Design review of the part built by this model. Coordinates are the model's own, in mm. A direction names the side the tool comes from. Round coordinates to 2 decimals unless told otherwise and drop trailing zeros. Loops run counter-clockwise (first coordinate to the right, second up) from the corner with the lowest first, then second, coordinate; pieces in that order, holes last. Notation, with made-up numbers: (7.25, 59) - (11.25, 59) arc R12 cw to (11.25, 69) - close; hole circle Ø1 at (43, 55). An arc over 180 degrees is marked (long way). Return JSON: item names as keys, results as strings. Group by question number.
(1) Clearance check with flat-ended pins moving along their axes: pin 1 (6 mm diameter, centred on x = -9.98, z = -5.76, fed in from +Y); pin 2 (1.6 mm diameter, centred on x = 9.99, z = 5.76, fed in from -Y); pin 3 (2 mm diameter, centred on x = 0, z = 11.53, fed in from +Y); pin 4 (5 mm diameter, centred on x = 2, z = -4.5, fed in from -Y). State where each tip first meets the part, or that it passes through.
(2) Wall thickness on L1, parallel to X at y = -1.35, z = 0; L2, parallel to X at y = -0.2, z = 5.75; L3, parallel to X at y = -1.55, z = 6: over which ranges is each line inside the solid? List them lowest first. Write a range as [from, to].
(3) For faces 5 (the cylindrical face through (0.709, 1.232, 9.816)), 6 (the cylindrical face through (-2.91, 0.13, -7.02)), 7 (the cylindrical face through (0.27, -0.81, 10.67)), list the 3-axis set-ups (+Z, -Z, +X, -X, +Y, -Y) from which the entire face can be reached by the end or side of a thin tool; tool diameter is ignored.
(4) The part is to be moulded in two halves that separate along Z. For faces 1 (the cylindrical face through (9.1, -0.8, -5.6)), 2 (the cylindrical face through (-9.1, -0.8, -5.6)), 3 (the cylindrical face through (0.66, 0.421, 14.985)), 4 (the flat face through (-3.5, 2.7, -6.4)), say which applies: pulls with the +Z half, pulls with the -Z half, needs draft (parallel to the pull), parting line crosses it, or undercut.
(5) We need section A-A, the plane y = -1.2. Write out the cut boundary in (x, z) (3 decimals).
(6) We need section B-B, the plane x = 0. Give the number of separate pieces and of enclosed holes in the cut face, and give its area (3 significant figures).
from build123d import *

# Parameters (mm, degrees)
SKETCH_1_R          = 15
SKETCH_1_R_2        = 7.1
SKETCH_1_R_3        = 1.85
EXTRUDE_1_DEPTH     = 2.7
EXTRUDE_START       = 1.8
SKETCH_2_R          = 15
SKETCH_2_R_2        = 7.1
SKETCH_2_R_3        = 0.9
EXTRUDE_2_DEPTH     = 1.8
SKETCH_3_R          = 7.6
CUT_EXTRUDE_1_DEPTH = 4.1
CHAMFER_1_SIZE      = 0.2
CHAMFER_2_SIZE      = 0.4


with BuildPart() as part:
    # 草图1 → 凸台-拉伸1 (new body)
    with BuildSketch(Plane(origin=(0, 0, 0), x_dir=(1, 0, 0), z_dir=(0, 1, 0))):
        with Locations(Location((0, 0, 0), (0, 0, 90))):
            Circle(SKETCH_1_R)
        with Locations(Location((0, 0, 0), (0, 0, 90))):
            Circle(SKETCH_1_R_2, mode=Mode.SUBTRACT)
        with Locations(Location((0, 11.525, 0), (0, 0, 90))):
            Circle(SKETCH_1_R_3, mode=Mode.SUBTRACT)
        with Locations(Location((9.980942779, 5.7625, 0), (0, 0, 90))):
            Circle(SKETCH_1_R_3, mode=Mode.SUBTRACT)
        with Locations(Location((9.980942779, -5.7625, 0), (0, 0, 90))):
            Circle(SKETCH_1_R_3, mode=Mode.SUBTRACT)
        with Locations(Location((0, -11.525, 0), (0, 0, 90))):
            Circle(SKETCH_1_R_3, mode=Mode.SUBTRACT)
        with Locations(Location((-9.980942779, -5.7625, 0), (0, 0, 90))):
            Circle(SKETCH_1_R_3, mode=Mode.SUBTRACT)
        with Locations(Location((-9.980942779, 5.7625, 0), (0, 0, 90))):
            Circle(SKETCH_1_R_3, mode=Mode.SUBTRACT)
    extrude(amount=EXTRUDE_1_DEPTH)

    # 草图2 → 凸台-拉伸2 (add)
    with BuildSketch(Plane(origin=(0, 0, 0), x_dir=(-1, 0, 0), z_dir=(0, -1, 0)).offset(EXTRUDE_START)):
        with Locations(Location((0, 0, 0), (0, 0, 90))):
            Circle(SKETCH_2_R)
        with Locations(Location((0, 0, 0), (0, 0, 90))):
            Circle(SKETCH_2_R_2, mode=Mode.SUBTRACT)
        with Locations(Location((0, 11.53, 0), (0, 0, 90))):
            Circle(SKETCH_2_R_3, mode=Mode.SUBTRACT)
        with Locations(Location((9.985272906, 5.765, 0), (0, 0, 90))):
            Circle(SKETCH_2_R_3, mode=Mode.SUBTRACT)
        with Locations(Location((9.985272906, -5.765, 0), (0, 0, 90))):
            Circle(SKETCH_2_R_3, mode=Mode.SUBTRACT)
        with Locations(Location((0, -11.53, 0), (0, 0, 90))):
            Circle(SKETCH_2_R_3, mode=Mode.SUBTRACT)
        with Locations(Location((-9.985272906, -5.765, 0), (0, 0, 90))):
            Circle(SKETCH_2_R_3, mode=Mode.SUBTRACT)
        with Locations(Location((-9.985272906, 5.765, 0), (0, 0, 90))):
            Circle(SKETCH_2_R_3, mode=Mode.SUBTRACT)
    extrude(amount=-EXTRUDE_2_DEPTH)

    # 草图3 → 切除-拉伸1 (cut)
    with BuildSketch(Plane(origin=(0, -1.8, 0), x_dir=(-1, 0, 0), z_dir=(0, -1, 0))):
        with Locations(Location((0, 0, 0), (0, 0, 90))):
            Circle(SKETCH_3_R)
    extrude(amount=-CUT_EXTRUDE_1_DEPTH, mode=Mode.SUBTRACT)

    # 倒角1
    chamfer_1_edges = [part.edges().sort_by_distance(p)[0] for p in [
        (9.980942779, 2.7, -3.9125),
        (9.980942779, 2.7, 7.6125),
        (0, 2.7, 13.375),
        (-9.980942779, 2.7, 7.6125),
        (-9.980942779, 2.7, -3.9125),
        (0, -1.8, 15),
        (0, -1.8, -10.63),
        (-9.985272906, -1.8, -4.865),
        (-9.985272906, -1.8, 6.665),
        (0, -1.8, 12.43),
        (9.985272906, -1.8, 6.665),
        (9.985272906, -1.8, -4.865),
        (0, 2.7, 15),
        (0, -1.8, 7.6),
        (0, 2.7, -9.675),
    ]]
    chamfer(chamfer_1_edges, length=CHAMFER_1_SIZE)

    # 倒角2
    chamfer_2_edges = [part.edges().sort_by_distance(p)[0] for p in [
        (0, 2.3, 7.6),
    ]]
    chamfer(chamfer_2_edges, length=CHAMFER_2_SIZE)


solid = part.part
Solutions:
{
 "1": {"pin 1": "y = 2.7", "pin 2": "through", "pin 3": "y = 0", "pin 4": "y = 2.08"},
 "2": {"L1": "[-15, -7.6], [7.6, 15]", "L2": "[-13.85, -10.89], [-9.09, -4.97], [4.97, 9.09], [10.89, 13.85]", "L3": "[-13.75, -10.85], [-9.12, -4.66], [4.66, 9.12], [10.85, 13.75]"},
 "3": {"face 5": "+Y", "face 6": "-Y", "face 7": "+Y, -Y"},
 "4": {"face 1": "undercut", "face 2": "undercut", "face 3": "parting line crosses it", "face 4": "needs draft"},
 "5": {"outline": "circle Ø30 at (0, 0); hole circle Ø1.8 at (-9.985, -5.765); hole circle Ø1.8 at (-9.985, 5.765); hole circle Ø15.2 at (0, 0); hole circle Ø1.8 at (0, -11.53); hole circle Ø1.8 at (0, 11.53); hole circle Ø1.8 at (9.985, -5.765); hole circle Ø1.8 at (9.985, 5.765)"},
 "6": {"separate pieces": "4", "enclosed holes": "0", "area": "40.4 mm^2"}
}
